Input: part model. Units: mm. Frame: model coordinates. Face numbers are marked on the shaded views. A direction names the side the tool comes from. Give positions to 0.01 mm unless a question says otherwise; leave off trailing zeros. Order: outer loops, then holes, each group sorted by start corner. A loop starts at its lowest first (then second) coordinate and runs counter-clockwise, first axis right, second up. Notation, with made-up numbers: (71.25, -8) - (106.25, -8) arc R35 cw to (106.25, 24) - close; hole circle Ø6 at (45.5, -21). An arc over 180 degrees is marked (long way). Use a Markdown table: item, result.
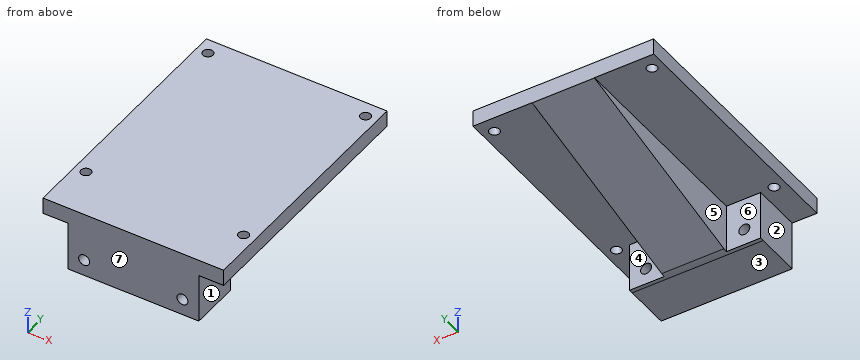
from build123d import *

# Parameters (mm, degrees)
SKETCH_1_W          = 65
SKETCH_1_H          = 100
EXTRUDE_1_DEPTH     = 5
SKETCH_3_W          = 65
SKETCH_3_H          = 15
EXTRUDE_2_DEPTH     = 15
SKETCH_4_R          = 1.675
CUT_EXTRUDE_1_DEPTH = 15
SKETCH_8_R          = 1.55
CUT_EXTRUDE_2_DEPTH = 15
EXTRUDE_4_DEPTH     = 19
SKETCH_10_W         = 12.51
SKETCH_10_H         = 20.752848232
SKETCH_10_H_2       = 21.550243719
CUT_EXTRUDE_3_DEPTH = 93.229333728
SKETCH_11_W         = 65
SKETCH_11_H         = 22.160800115
CUT_EXTRUDE_4_DEPTH = 10
FILLET_START        = -21
FILLET_1_DEPTH      = 42
SKETCH_12_W         = 13.248565373
SKETCH_12_H         = 85.777871489
SKETCH_12_W_2       = 8.637190958
SKETCH_12_H_2       = 86.586054809
CUT_EXTRUDE_6_DEPTH = 10


with BuildPart() as part:
    # 草图1 → 凸台-拉伸1 (new body)
    with BuildSketch(Plane.XY):
        Rectangle(SKETCH_1_W, SKETCH_1_H)
    extrude(amount=EXTRUDE_1_DEPTH)

    # 草图3 → 凸台-拉伸2 (add)
    with BuildSketch(Plane(origin=(0, 0, 0), x_dir=(-1, 0, 0), z_dir=(0, 0, -1))):
        with Locations((0, -42.5)):
            Rectangle(SKETCH_3_W, SKETCH_3_H)
    extrude(amount=EXTRUDE_2_DEPTH)

    # 草图4 → 切除-拉伸1 (cut)
    with BuildSketch(Plane(origin=(0, -35, 0), x_dir=(1, 0, 0), z_dir=(0, 1, 0))):
        with Locations(Location((-14.99, 10, 0), (0, 0, 270))):
            Circle(SKETCH_4_R)
        with Locations(Location((14.99, 10, 0), (0, 0, 270))):
            Circle(SKETCH_4_R)
    extrude(amount=-CUT_EXTRUDE_1_DEPTH, mode=Mode.SUBTRACT)

    # 草图8 → 切除-拉伸2 (cut)
    with BuildSketch(Plane.XY.offset(5)):
        with Locations((-24.05, 23.1)):
            Circle(SKETCH_8_R)
        with Locations((24.05, 23.1)):
            Circle(SKETCH_8_R)
        with Locations((-24.05, -35)):
            Circle(SKETCH_8_R)
        with Locations((24.05, -35)):
            Circle(SKETCH_8_R)
    extrude(amount=-CUT_EXTRUDE_2_DEPTH, mode=Mode.SUBTRACT)

    # 草图9 → 凸台-拉伸4 (add)
    with BuildSketch(Plane(origin=(9.5, 0, 0), x_dir=(0, 0, -1), z_dir=(1, 0, 0))):
        Polygon((15, -35), (0, -35), (0, 28.153160969), align=None)
    extrude(amount=-EXTRUDE_4_DEPTH)

    # 草图10 → 切除-拉伸3 (cut, through all)
    with BuildSketch(Plane(origin=(0, -35, 0), x_dir=(1, 0, 0), z_dir=(0, 1, 0))):
        with Locations((26.245, 10.376424116)):
            Rectangle(SKETCH_10_W, SKETCH_10_H)
        with Locations((-26.245, 10.77512186)):
            Rectangle(SKETCH_10_W, SKETCH_10_H_2)
    extrude(amount=-CUT_EXTRUDE_3_DEPTH, mode=Mode.SUBTRACT)

    # 草图11 → 切除-拉伸4 (cut)
    with BuildSketch(Plane.XY.offset(5)):
        with Locations((0, 38.919599942)):
            Rectangle(SKETCH_11_W, SKETCH_11_H)
    extrude(amount=-CUT_EXTRUDE_4_DEPTH, mode=Mode.SUBTRACT)

    # 圆角1: read off the stored shape, not the designer's step
    # 圆角1 outline → 圆角1 (cut)
    with BuildSketch(Plane.YZ.offset(FILLET_START)):
        with BuildLine():
            Line((-36.171296068, -15), (-35, -15))
            Line((-35, -15), (-33.860407805, -14.729326566))
            add(Edge.make_bspline(
                [(-33.860407805, -14.729326566), (-34.0852258, -14.782724842), (-34.31196566, -14.829719593), (-34.540261945, -14.87017776), (-34.769736346, -14.904008746), (-35.233444691, -14.958699176), (-35.467701672, -14.979373092), (-35.702365681, -14.993139997), (-35.937031343, -15), (-36.171296068, -15)],
                knots=[0.503429998, 0.503429998, 0.503429998, 0.503429998, 0.503429998, 0.503429998, 1, 1, 1, 1, 1.503429998, 1.503429998, 1.503429998, 1.503429998, 1.503429998, 1.503429998], degree=5, weights=[1, 1, 0.99999889, 0.999998883, 1, 1, 0.999998819, 0.999998827, 1, 1]))
        make_face()
    extrude(amount=FILLET_1_DEPTH, mode=Mode.SUBTRACT)

    # 草图12 → 切除-拉伸6 (cut)
    with BuildSketch(Plane(origin=(0, 0, 0), x_dir=(-1, 0, 0), z_dir=(0, 0, -1))):
        with Locations((-34.174282686, -10.092547721)):
            Rectangle(SKETCH_12_W, SKETCH_12_H)
        with Locations((31.868595479, -11.75852662)):
            Rectangle(SKETCH_12_W_2, SKETCH_12_H_2)
    extrude(amount=-CUT_EXTRUDE_6_DEPTH, mode=Mode.SUBTRACT)


solid = part.part
1. Section query C-C (z = -10.5). Return loops of the section in (x, y), then the cut area to 3 significant figures.
Response:
| item | result |
|---|---|
| outline | (-19.99, -50) - (-16.59, -50) - (-16.59, -35) - (-19.99, -35) - close; (-13.39, -50) - (13.39, -50) - (13.39, -35) - (9.5, -35) - (9.5, -16.05) - (-9.5, -16.05) - (-9.5, -35) - (-13.39, -35) - close; (16.59, -50) - (19.99, -50) - (19.99, -35) - (16.59, -35) - close |
| area | 864 mm^2 |
2. Section query D-D (y = -19.5). Return loops of the section in (x, z).
Response:
| item | result |
|---|---|
| outline | (-27.55, 0) - (-9.5, 0) - (-9.5, -11.32) - (9.5, -11.32) - (9.5, 0) - (27.55, 0) - (27.55, 5) - (-27.55, 5) - close |
3. Section query A-A (x = -24.05). Return loops of the section in (y, z).
Response:
| item | result |
|---|---|
| outline | (-50, 0) - (-36.55, 0) - (-36.55, 5) - (-50, 5) - close; (-33.45, 0) - (21.55, 0) - (21.55, 5) - (-33.45, 5) - close; (24.65, 0) - (27.84, 0) - (27.84, 5) - (24.65, 5) - close |
4. Material intervals for line 1 along Y through (x, z) = (24.05, 3.6); line 2 along Y through (x, z) = (14, -6); line 3 along X through (y, z) = (-42, -12.75), sorted ascending.
Response:
| item | result |
|---|---|
| line 1 | y = -50 to -36.55, -33.45 to 21.55, 24.65 to 27.84 |
| line 2 | y = -50 to -35 |
| line 3 | x = -19.99 to 19.99 |
5. Mould query, pull axis Y, two halves, no side actions, for the marked faces 5, 6 and 7. Classes: pulls with the +Y half, pulls with the -Y half, needs draft (parallel to the pull), parting line crosses it, or undercut.
Response:
| item | result |
|---|---|
| face 5 | needs draft |
| face 6 | pulls with the +Y half |
| face 7 | pulls with the -Y half |
6. Section query B-B (y = 23.1). Return loops of the section in (x, z).
Response:
| item | result |
|---|---|
| outline | (-27.55, 0) - (-25.6, 0) - (-25.6, 5) - (-27.55, 5) - close; (-22.5, 0) - (-9.5, 0) - (-9.5, -1.2) - (9.5, -1.2) - (9.5, 0) - (22.5, 0) - (22.5, 5) - (-22.5, 5) - close; (25.6, 0) - (27.55, 0) - (27.55, 5) - (25.6, 5) - close |
7. Pin query (flat end, axial travel): pin 1 (11.5 mm diameter, centred on x = -17, z = -6, fed in from +Y); pin 2 (7.5 mm diameter, centred on y = -2, z = -10.5, fed in from -X); pin 3 (20 mm diameter, centred on x = -16, y = -20, fed in from -Z). Return the tip coordinate at first contact, or that it passes through.
Response:
| item | result |
|---|---|
| pin 1 | stops at y = -35 |
| pin 2 | stops at x = -9.5 |
| pin 3 | stops at z = -13.24 |
8. Set-up query: the marked faces 1, 2, 3 and 4. Return all of +Z, -Z, +X, -X, +Y, -Y with unobstructed straight access to the full face (end or side cutting, diameter ignored); none if empty.
Response:
| item | result |
|---|---|
| face 1 | -Z, +X, +Y, -Y |
| face 2 | -Z, -X, +Y, -Y |
| face 3 | -Z, +X, -X, +Y, -Y |
| face 4 | -Z, +X, +Y |
